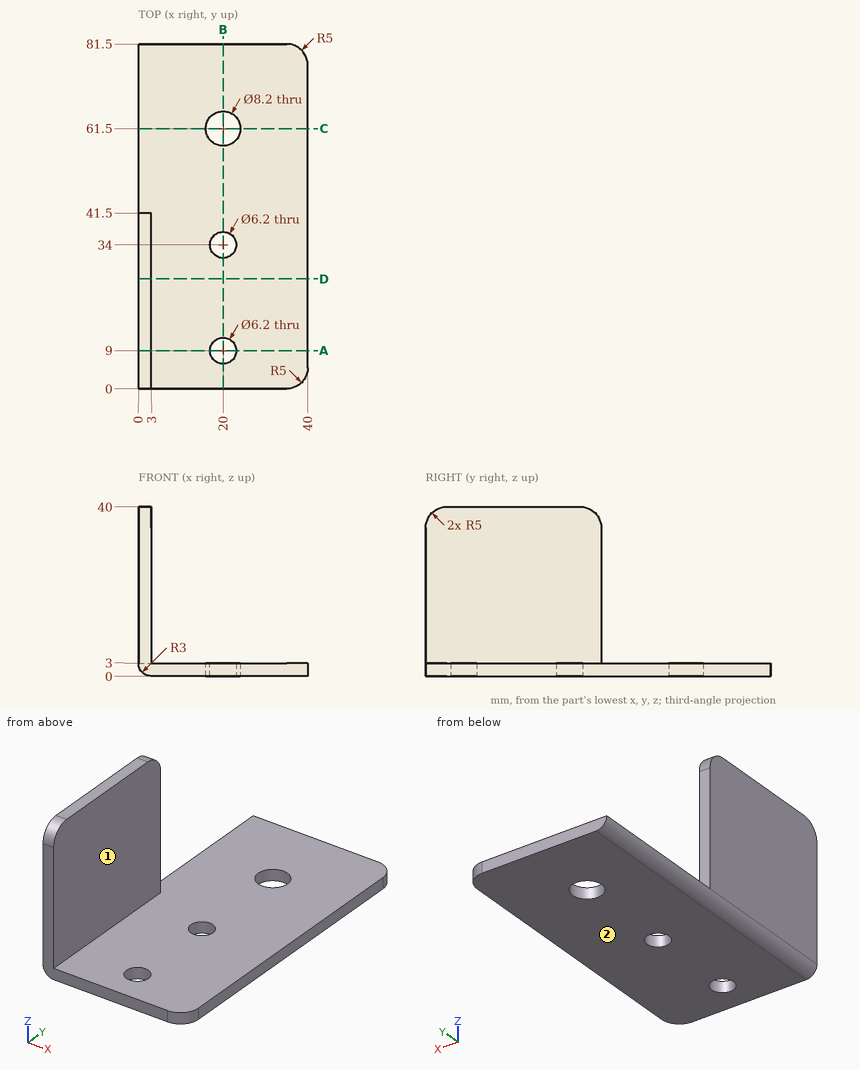
The drawing under review shows one solid part. Ordinate dimensions are in mm from its lowest x, y, z. A direction names the side the tool comes from. Round coordinates to 2 decimals unless told otherwise and drop trailing zeros. Write each loop counter-clockwise with the first axis right and the second up, starting at its lowest first coordinate (ties: lowest second). Pieces come first, ordered by that corner, then holes. Notation, with made-up numbers: (-31, 21) - (11, 21) arc R24 cw to (11, 42) - close; hole circle Ø8 at (5.5, 2.25). An arc over 180 degrees is marked (long way). Use one line per item in the form item = value.
Q1. Insertion check: pin 1 Ø6 at (x, y) = (26, 70) entering from +Z; pin 2 Ø5 at (y, z) = (33.5, 32) entering from +X; pin 3 Ø3.5 at (x, z) = (1, 22.5) entering from +Y. Each pin has a flat end and moves straight along its axis. Give the tip position at first contact, or say it passes through.
Answer key:
pin_1 = 3
pin_2 = 3
pin_3 = 41.5
Q2. Consider section A-A (y = 9). State the section outline as (x, z) points, and give its area (3 significant figures).
Answer key:
outline = (0, 3) arc R3 ccw to (3, 0) - (16.9, 0) - (16.9, 3) - (3, 3) - (3, 40) - (0, 40) - close; (23.1, 0) - (40, 0) - (40, 3) - (23.1, 3) - close
area = 210 mm2
Q3. For line 1 (Y direction, x = 20, z = 1); line 2 (Z direction, x = 35, y = 40), list the stretches that pass through material, from the lowest coordinate up. Write a range as [from, to].
Answer key:
line_1 = [0, 5.9], [12.1, 30.9], [37.1, 57.4], [65.6, 81.5]
line_2 = [0, 3]
Q4. Consider section B-B (x = 20). State the section outline as (y, z) points.
Answer key:
outline = (0, 0) - (5.9, 0) - (5.9, 3) - (0, 3) - close; (12.1, 0) - (30.9, 0) - (30.9, 3) - (12.1, 3) - close; (37.1, 0) - (57.4, 0) - (57.4, 3) - (37.1, 3) - close; (65.6, 0) - (81.5, 0) - (81.5, 3) - (65.6, 3) - close
Q5. Consider section D-D (y = 26). State the section outline as (x, z) points.
Answer key:
outline = (0, 3) arc R3 ccw to (3, 0) - (40, 0) - (40, 3) - (3, 3) - (3, 40) - (0, 40) - close
Q6. Tool access review of the marked faces 1 and 2: name each direction out of +Z, -Z, +X, -X, +Y, -Y from which nothing blocks a thin tool from reaching the whole face with its end or side.
Answer key:
face_1 = +Z, +X, +Y, -Y
face_2 = -Z, +X, -X, +Y, -Y
Q7. Consider section C-C (y = 61.5). State the section outline as (x, z) points, and give its area (3 significant figures).
Answer key:
outline = (0, 3) arc R3 ccw to (3, 0) - (15.9, 0) - (15.9, 3) - close; (24.1, 0) - (40, 0) - (40, 3) - (24.1, 3) - close
area = 93.5 mm2
